Part model, mm, in its own coordinate system. Coordinates: 2 decimals unless noted, no trailing zeros. Order: outer loops, then holes, each group sorted by start corner. A loop starts at its lowest first (then second) coordinate and runs counter-clockwise, first axis right, second up.
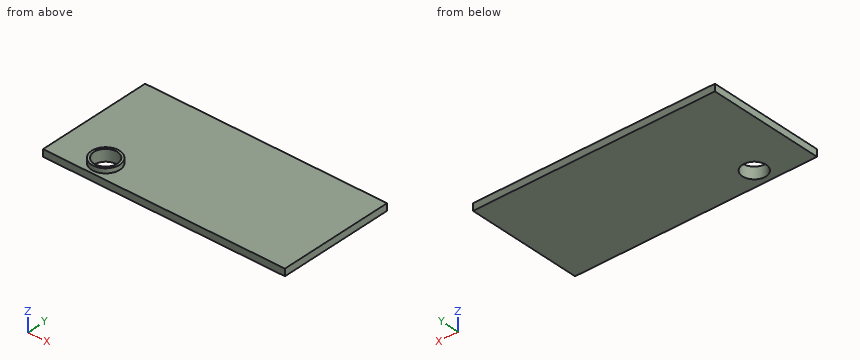
from build123d import *

# Parameters (mm, degrees)
F0_W     = 1321.300506
F0_H     = 635.08135
F0_R     = 64.413244
F1_DEPTH = 38.1
F2_R     = 77.113234
F2_R_2   = 64.413244
F3_DEPTH = 25.4


with BuildPart() as f1:
    # F0 (on Top) → F1 (new body)
    with BuildSketch(Plane.XY):
        Rectangle(F0_W, F0_H)
        with Locations((-401.148856, -223.188221)):
            Circle(F0_R, mode=Mode.SUBTRACT)
    extrude(amount=F1_DEPTH)

    # F2 (on face) → F3 (join)
    with BuildSketch(Plane.XY.offset(38.1)):
        with Locations((-401.148856, -223.188221)):
            Circle(F2_R)
        with Locations((-401.148856, -223.188221)):
            Circle(F2_R_2, mode=Mode.SUBTRACT)
    extrude(amount=F3_DEPTH)


solid = f1.part
Q1. Pin check, flat tips, straight feed: pin 1 Ø1 at (x, y) = (391.5, -127.5) entering from -Z; pin 2 Ø12 at (x, y) = (525.5, 100.5) entering from +Z. Stop position of each tip, or through.
Results list:
pin 1: stops at z = 0
pin 2: stops at z = 38.1
Q2. Cut at C-C on x = 126. Write the cut outline in (y, z).
Results list:
outline: (-317.54, 0) - (317.54, 0) - (317.54, 38.1) - (-317.54, 38.1) - close
Q3. Cut at B-B on z = 22. Write the cut outline in (x, y), and give its area (3 significant figures).
Results list:
outline: (-660.65, -317.54) - (660.65, -317.54) - (660.65, 317.54) - (-660.65, 317.54) - close; hole circle Ø128.83 at (-401.15, -223.19)
area: 826,000 mm2
Q4. Cut at D-D on y = -12. Write the cut outline in (x, z), and give its area (3 significant figures).
Results list:
outline: (-660.65, 0) - (660.65, 0) - (660.65, 38.1) - (-660.65, 38.1) - close
area: 50,300 mm2
Q5. Wall check: line 1 along Z through (x, y) = (48, -162); line 2 along Y through (x, z) = (-440.5, 60); line 3 along X through (y, z) = (-263, 10). Give the ranges that are in metal, low to high.
Results list:
line 1: z = 0 to 38.1
line 2: y = -289.51 to -274.18, -172.19 to -156.87
line 3: x = -660.65 to -451.79, -350.51 to 660.65
Q6. Cut at A-A on y = -204. Write the cut outline in (x, z).
Results list:
outline: (-660.65, 0) - (-462.64, 0) - (-462.64, 63.5) - (-475.84, 63.5) - (-475.84, 38.1) - (-660.65, 38.1) - close; (-339.66, 0) - (660.65, 0) - (660.65, 38.1) - (-326.46, 38.1) - (-326.46, 63.5) - (-339.66, 63.5) - close
